Input: dimensioned drawing with shaded views. Units: mm. Origin: part minimum x, y, z. A direction names the side the tool comes from. Coordinates: 2 decimals unless noted, no trailing zeros. Order: outer loops, then holes, each group sorted by start corner. A loop starts at its lowest first (then second) coordinate and runs counter-clockwise, first axis right, second up. Notation, with made-up numbers: (22, -4) - (59, -4) arc R5 ccw to (59, 3) - close; hole circle Ø4 at (57.25, 45.5). An arc over 180 degrees is marked (long way). One line per question, with ' | ' between items. Start each with the question number.
(1) Section C-C (z = 8.75). Return the cut outline in (x, y), then the cut area to 3 significant figures.
(2) Line query: line 1 along Y through (x, z) = (59.7, 14); line 2 along X through (y, z) = (64.5, 2.75); line 3 along Z through (x, y) = (45, 10.5). Output: solid intervals per line, ascending.
(3) Section A-A (z = 12.5). Return the cut outline in (x, y), then the cut area to 3 significant figures.
(4) Section B-B (y = 55). Return the cut outline in (x, z), then the cut area to 3 significant figures.
(5) Access query for the marked faces 1 and 2. Directions: +Z, -Z, +X, -X, +Y, -Y. A direction counts if a zero-diameter tool reaches every point of the face in a straight line with its end or side. Return the directions, or none.
(6) Section D-D (x = 9). Return the cut outline in (y, z).
(7) Contact query for flat-ended pins moving along their axis: P1, Ø8, axis at x = 23.5, y = 58, coming from the +Z side; P2, Ø12, axis at x = 53.5, y = 10, coming from the +Z side; P3, Ø4, axis at y = 55, z = 14, coming from the +X side. Output: stop coordinate, or through.
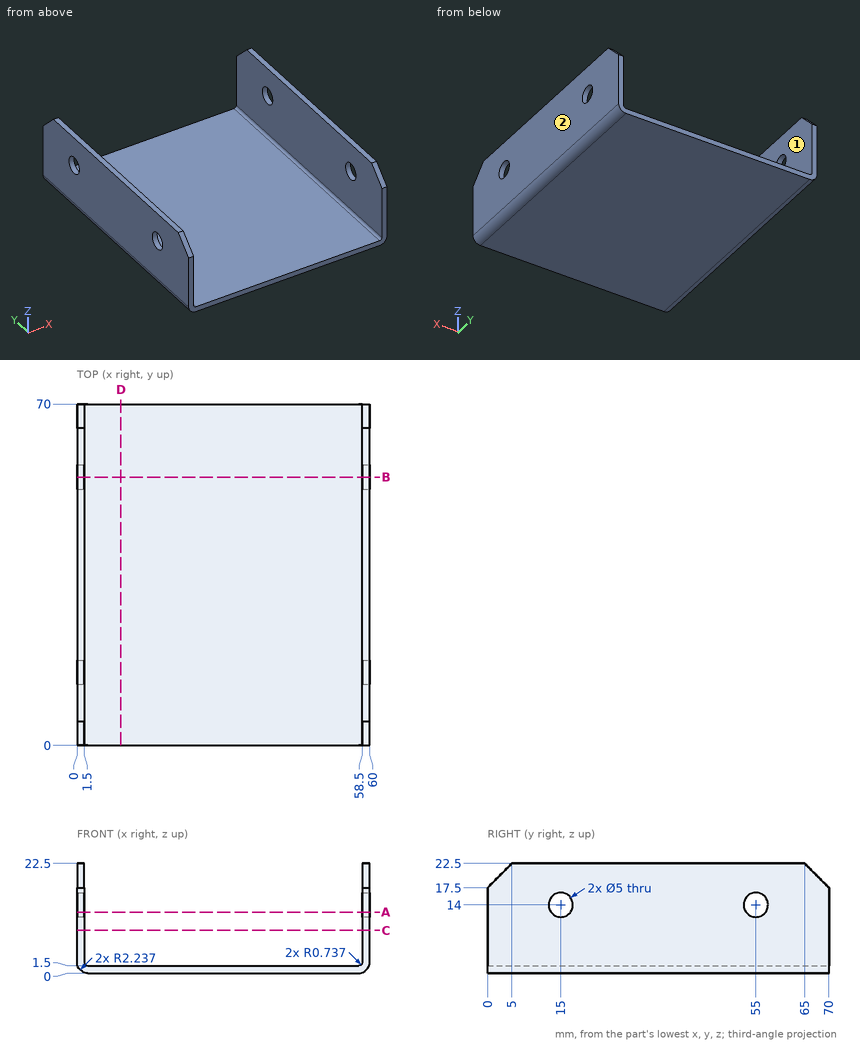
Response values:
1) outline: (0, 0) - (1.5, 0) - (1.5, 70) - (0, 70) - close; (58.5, 0) - (60, 0) - (60, 70) - (58.5, 70) - close | area: 210 mm²
2) line 1: y = 0 to 12.5, 17.5 to 52.5, 57.5 to 70 | line 2: x = 0 to 1.5, 58.5 to 60 | line 3: z = 0 to 1.5
3) outline: (0, 0) - (1.5, 0) - (1.5, 13) - (0, 13) - close; (0, 17) - (1.5, 17) - (1.5, 53) - (0, 53) - close; (0, 57) - (1.5, 57) - (1.5, 70) - (0, 70) - close; (58.5, 0) - (60, 0) - (60, 13) - (58.5, 13) - close; (58.5, 17) - (60, 17) - (60, 53) - (58.5, 53) - close; (58.5, 57) - (60, 57) - (60, 70) - (58.5, 70) - close | area: 186 mm²
4) outline: (0, 2.24) arc R2.24 ccw to (2.24, 0) - (57.76, 0) arc R2.24 ccw to (60, 2.24) - (60, 11.5) - (58.5, 11.5) - (58.5, 2.24) arc R0.74 cw to (57.76, 1.5) - (2.24, 1.5) arc R0.74 cw to (1.5, 2.24) - (1.5, 11.5) - (0, 11.5) - close; (0, 16.5) - (1.5, 16.5) - (1.5, 22.5) - (0, 22.5) - close; (58.5, 16.5) - (60, 16.5) - (60, 22.5) - (58.5, 22.5) - close | area: 136 mm²
5) face 1: +Z, +Y, -Y | face 2: +Z, -Z, +X, +Y, -Y
6) outline: (0, 0) - (70, 0) - (70, 1.5) - (0, 1.5) - close
7) P1: stops at z = 1.5 | P2: stops at z = 22.5 | P3: passes through
